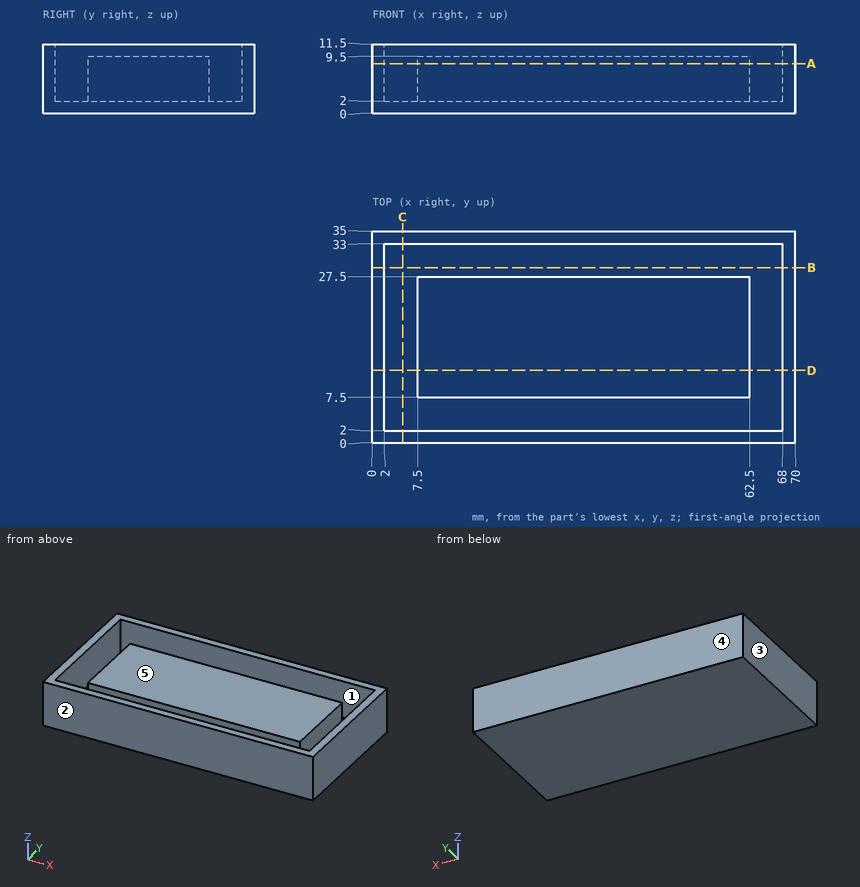
Print and shaded views of the part. All mm, measured from the part's lowest x, y and z. A direction names the side the tool comes from. Give positions to 0.01 mm unless a question says otherwise; leave off trailing zeros. Loops run counter-clockwise (first coordinate to the right, second up) from the corner with the lowest first, then second, coordinate; pieces in that order, holes last. Notation, with made-up numbers: (73, 9) -> (92, 9) arc R15 ccw to (92, 21) -> close; hole circle Ø3 at (-12.5, 24). An arc over 180 degrees is marked (long way). Answer in a Markdown table with one row per item.
Item 1: Slice it at A-A on z = 8.25. Write the cut outline in (x, y), plus the area to 3 significant figures.
Findings below:
| item | result |
|---|---|
| outline | (0, 0) -> (70, 0) -> (70, 35) -> (0, 35) -> close; (7.5, 7.5) -> (62.5, 7.5) -> (62.5, 27.5) -> (7.5, 27.5) -> close; hole (2, 2) -> (68, 2) -> (68, 33) -> (2, 33) -> close |
| area | 1,500 mm² |
Item 2: Slice it at C-C on x = 5. Write the cut outline in (y, z).
Findings below:
| item | result |
|---|---|
| outline | (0, 0) -> (35, 0) -> (35, 11.5) -> (33, 11.5) -> (33, 2) -> (2, 2) -> (2, 11.5) -> (0, 11.5) -> close |
Item 3: Slice it at D-D on y = 12. Write the cut outline in (x, z).
Findings below:
| item | result |
|---|---|
| outline | (0, 0) -> (70, 0) -> (70, 11.5) -> (68, 11.5) -> (68, 2) -> (62.5, 2) -> (62.5, 9.5) -> (7.5, 9.5) -> (7.5, 2) -> (2, 2) -> (2, 11.5) -> (0, 11.5) -> close |
Item 4: Tool access for the marked faces 1 and 2: list every direction of +Z, -Z, +X, -X, +Y, -Y with a clear straight run to the whole face (end or side of a thin tool).
Findings below:
| item | result |
|---|---|
| face 1 | +Z |
| face 2 | +Z, -Z, +X, -X, -Y |
Item 5: Flat gauge pin, fed straight in: P1, Ø1, axis at x = 44, y = 8.5, coming from the +Z side. Where does the tip first touch, or does it go through?
Findings below:
| item | result |
|---|---|
| P1 | stops at z = 9.5 |
Item 6: Probe line 1 along Y through (x, z) = (34, 4); line 2 along X through (y, z) = (15, 8); line 3 along Y through (x, z) = (67, 8). List the from-to ranges inside material, lowest first. Write a range as [from, to].
Findings below:
| item | result |
|---|---|
| line 1 | y = [0, 2], [7.5, 27.5], [33, 35] |
| line 2 | x = [0, 2], [7.5, 62.5], [68, 70] |
| line 3 | y = [0, 2], [33, 35] |
Item 7: Slice it at B-B on y = 29. Write the cut outline in (x, z), plus the area to 3 significant figures.
Findings below:
| item | result |
|---|---|
| outline | (0, 0) -> (70, 0) -> (70, 11.5) -> (68, 11.5) -> (68, 2) -> (2, 2) -> (2, 11.5) -> (0, 11.5) -> close |
| area | 178 mm² |
Item 8: Mould opens along X. For the marked faces 3, 4 and 5 say: pulls with the +X half, pulls with the -X half, needs draft (parallel to the pull), parting line crosses it, or undercut.
Findings below:
| item | result |
|---|---|
| face 3 | pulls with the -X half |
| face 4 | needs draft |
| face 5 | undercut |
